```python
from build123d import *

# Parameters (mm, degrees)
SKETCH1_R           = 4.45
BOSS_EXTRUDE1_DEPTH = 10
BOSS_EXTRUDE2_START = 10.1
SKETCH2_W           = 60
SKETCH2_H           = 10
BOSS_EXTRUDE2_DEPTH = 109.8
BOSS_EXTRUDE3_DEPTH = 7.5
FILLET1_R           = 10
FILLET2_R           = 10


with BuildPart() as part:
    # Sketch1 → Boss-Extrude1 (new body)
    with BuildSketch(Plane.XY):
        with BuildLine():
            Line((62.029952175, 0), (119.9, 0))
            Line((119.9, 0), (119.9, 28.94))
            ThreePointArc((119.9, 28.94), (116.971067812, 36.011067812), (109.9, 38.94))
            Line((109.9, 38.94), (100, 38.94))
            ThreePointArc((100, 38.94), (80.1, 58.84), (100, 78.74))
            Line((100, 78.74), (103.295753204, 78.74))
            ThreePointArc((103.295753204, 78.74), (110.366821016, 81.668932188), (113.295753204, 88.74))
            Line((113.295753204, 88.74), (113.295753204, 97.89474782))
            ThreePointArc((113.295753204, 97.89474782), (108.902354922, 108.501349538), (98.295753204, 112.89474782))
            Line((98.295753204, 112.89474782), (31.704246796, 112.89474782))
            ThreePointArc((31.704246796, 112.89474782), (21.097645078, 108.501349538), (16.704246796, 97.89474782))
            Line((16.704246796, 97.89474782), (16.704246796, 88.74))
            ThreePointArc((16.704246796, 88.74), (19.633178984, 81.668932188), (26.704246796, 78.74))
            Line((26.704246796, 78.74), (30, 78.74))
            ThreePointArc((30, 78.74), (49.9, 58.84), (30, 38.94))
            Line((30, 38.94), (20.1, 38.94))
            ThreePointArc((20.1, 38.94), (13.028932188, 36.011067812), (10.1, 28.94))
            Line((10.1, 28.94), (10.1, 0))
            Line((10.1, 0), (62.029952175, 0))
        make_face()
        with Locations((30, 30.24)):
            Circle(SKETCH1_R, mode=Mode.SUBTRACT)
        with Locations((30, 87.44)):
            Circle(SKETCH1_R, mode=Mode.SUBTRACT)
        with Locations((100, 30.24)):
            Circle(SKETCH1_R, mode=Mode.SUBTRACT)
        with Locations((100, 87.44)):
            Circle(SKETCH1_R, mode=Mode.SUBTRACT)
    extrude(amount=-BOSS_EXTRUDE1_DEPTH)

    # Sketch2 → Boss-Extrude2 (add)
    with BuildSketch(Plane(origin=(0, 0, 0), x_dir=(0, 0, -1), z_dir=(1, 0, 0)).offset(BOSS_EXTRUDE2_START)):
        with Locations((40, 5)):
            Rectangle(SKETCH2_W, SKETCH2_H)
    extrude(amount=BOSS_EXTRUDE2_DEPTH)

    # Sketch3 → Boss-Extrude3 (add, symmetric)
    with BuildSketch(Plane.ZY.offset(-65)):
        Polygon((-10, 97.89474782), (-10, 10), (-56.427715737, 10), align=None)
    extrude(amount=BOSS_EXTRUDE3_DEPTH, both=True)

    # Fillet1
    fillet1_edges = [part.edges().sort_by_distance(p)[0] for p in [
        (72.5, 10, -33.213857868),
    ]]
    fillet(fillet1_edges, radius=FILLET1_R)

    # Fillet2
    fillet2_edges = [part.edges().sort_by_distance(p)[0] for p in [
        (57.5, 10, -33.213857868),
    ]]
    fillet(fillet2_edges, radius=FILLET2_R)


solid = part.part
```
Design review of the part built by this model. Coordinates are the model's own, in mm. A direction names the side the tool comes from. Give positions to 0.01 mm unless a question says otherwise; leave off trailing zeros. Order: outer loops, then holes, each group sorted by start corner. A loop starts at its lowest first (then second) coordinate and runs counter-clockwise, first axis right, second up. Notation, with made-up numbers: M 35,-35.5 L 46,-35.5 A12 ccw 46,-21.5 Z; hole C 44.25,53 d6. An arc over 180 degrees is marked long. One line per question, with ' | ' between items. Start each with the question number.
Q1. We need section A-A (y = 86). Write out the cut boundary in (x, z).
Q2. The part is to be moulded in two halves that separate along Y. For faces 5 (the face through (19.6, 81.7, -4.9)), 6 (the face through (64, 0, -35)), 7 (the face through (119.9, 8, -27)), 8 (the face through (75.51, 12.85, -33.54)), say which applies: +Y half, -Y half, draft (parallel to the pull), parting line (faces both ways), or undercut.
Q3. For L1, parallel to Y at x = 100, z = -7; L2, parallel to X at y = 30, z = -5; L3, parallel to X at y = 36, z = -37, list the stretches that pass through material, from the lowest coordinate up. Write a range as [from, to].
Q4. We need section D-D (y = 58). Write out the cut boundary in (x, z), plus the area to 3 significant figures.
Q5. Machinability: for faces 1 (the face through (28, 78.74, -5)), 2 (the face through (113.296, 93, -5)), 3 (the face through (72.5, 42, -21)), 4 (the face through (102, 78.74, -5)), which of the approach directions +Z, -Z, +X, -X, +Y, -Y give a long, thin tool a straight path to every point of the face, cutting with its end or side? Answer none if there is none.
Q6. For pin 1 Ø5 at (x, z) = (90, -37) entering from +Y; pin 2 Ø10 at (y, z) = (94.5, -6) entering from +X; pin 3 Ø1.5 at (y, z) = (18, -25) entering from -X; pin 4 Ø7 at (x, y) = (30, 87.44) entering from +Z, all flat-tipped, find the tip position at first contact; note any pin that passes through.
Q7. We need section B-B (x = 23). Write out the cut boundary in (y, z).
Q8. We need section C-C (z = -38). Write out the cut boundary in (x, y), plus the area to 3 significant figures.
Returned:
1) outline: M 17.09,-10 L 25.79,-10 L 25.79,0 L 17.09,0 Z; M 34.21,-10 L 57.5,-10 L 57.5,-16.28 L 72.5,-16.28 L 72.5,-10 L 95.79,-10 L 95.79,0 L 34.21,0 Z; M 104.21,-10 L 112.91,-10 L 112.91,0 L 104.21,0 Z
2) face 5: undercut | face 6: -Y half | face 7: draft | face 8: +Y half
3) L1: [0, 25.79], [34.69, 38.94], [78.74, 82.99], [91.89, 112.8] | L2: [10.16, 25.56], [34.44, 95.56], [104.44, 119.84] | L3: [57.5, 72.5]
4) outline: M 49.88,-10 L 57.5,-10 L 57.5,-31.07 L 72.5,-31.07 L 72.5,-10 L 80.12,-10 L 80.12,0 L 49.88,0 Z | area: 618 mm2
5) face 1: +Z, -Z, -X | face 2: +Z, -Z, +X, +Y | face 3: -Z, +X, +Y | face 4: +Z, -Z, +X
6) pin 1: y = 10 | pin 2: x = 113.3 | pin 3: x = 57.11 | pin 4: through
7) outline: M 0,-70 L 10,-70 L 10,-10 L 38.94,-10 L 38.94,0 L 0,0 Z; M 79.45,-10 L 110.11,-10 L 110.11,0 L 79.45,0 Z
8) outline: M 10.1,0 L 119.9,0 L 119.9,10 L 82.5,10 A10 cw 72.5,20 L 72.5,44.89 L 57.5,44.89 L 57.5,20 A10 cw 47.5,10 L 10.1,10 Z | area: 1,660 mm2
